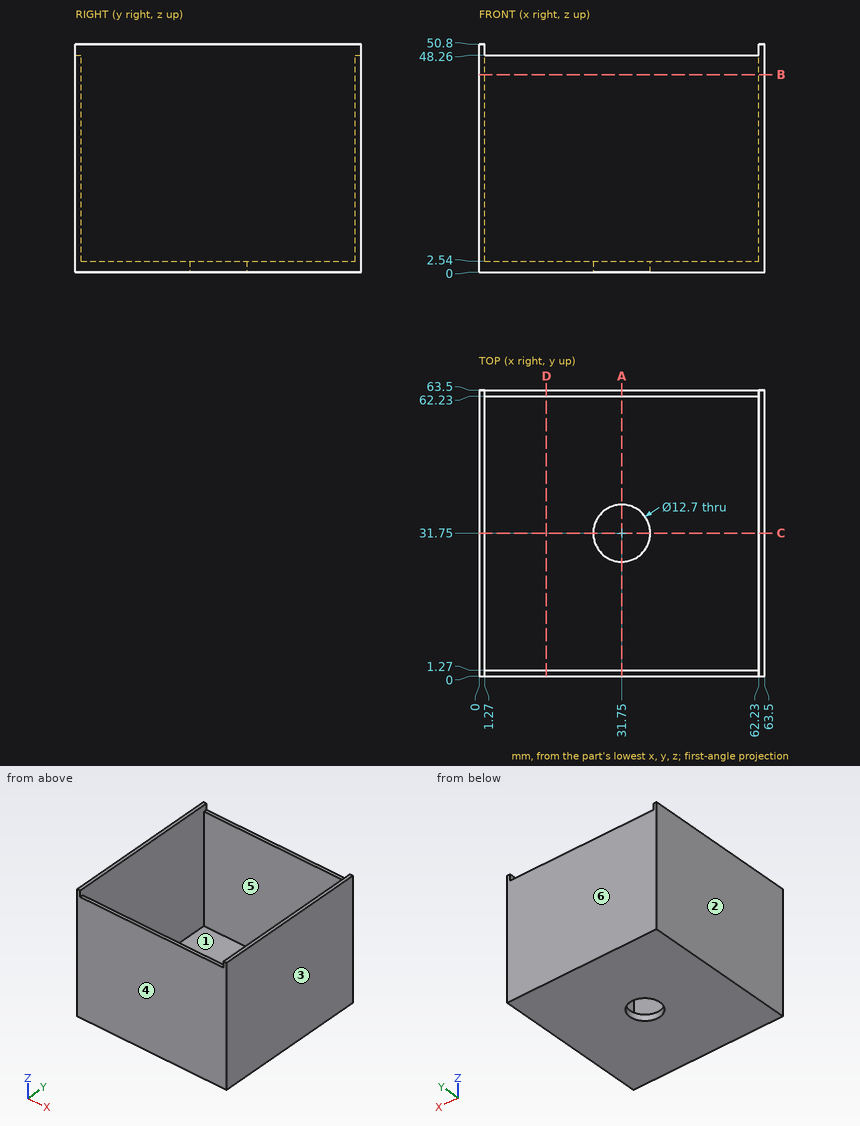
Job drawing, mm, ordinate dimensions from the low corner. One solid piece. A direction names the side the tool comes from. Coordinates: 2 decimals unless noted, no trailing zeros. Order: outer loops, then holes, each group sorted by start corner. A loop starts at its lowest first (then second) coordinate and runs counter-clockwise, first axis right, second up. Notation, with made-up numbers: (79, 38.25) - (91, 38.25) arc R22 ccw to (91, 74.25) - close; hole circle Ø6 at (50, 11). An arc over 180 degrees is marked (long way). Return JSON: item names as keys, results as strings. Group by question number.
1) Saw through at C-C, the plane y = 31.75. Write the cut outline in (x, z), plus the area to 3 significant figures.
2) Flat gauge pins, fed straight in: P1, Ø1, axis at x = 39.5, y = 0.5, coming from the +Z side; P2, Ø1.5, axis at x = 39, y = 15.5, coming from the +Z side; P3, Ø10, axis at x = 31.75, y = 31.75, coming from the +Z side. Where does each tip first touch, or does it go through?
3) Probe line 1 (Y direction, x = 7, z = 45.5); line 2 (Y direction, x = 31.75, z = 2.05). List the from-to ranges inside material, lowest first. Write a range as from..to.
4) Saw through at B-B, the plane z = 44. Write the cut outline in (x, y).
5) Mould opens along X. For the marked faces 1, 2, 3 and 4 say: released by +X, released by -X, zero draft, split by the parting line, or undercut.
6) Saw through at D-D, the plane x = 15. Write the cut outline in (y, z).
7) Saw through at A-A, the plane x = 31.75. Write the cut outline in (y, z).
8) Tool access for the marked faces 5 and 6: list every direction of +Z, -Z, +X, -X, +Y, -Y with a clear straight run to the whole face (end or side of a thin tool).
Values found:
{
 "1": {"outline": "(0, 0) - (25.4, 0) - (25.4, 2.54) - (1.27, 2.54) - (1.27, 50.8) - (0, 50.8) - close; (38.1, 0) - (63.5, 0) - (63.5, 50.8) - (62.23, 50.8) - (62.23, 2.54) - (38.1, 2.54) - close", "area": "252 mm²"},
 "2": {"P1": "stops at z = 48.26", "P2": "stops at z = 2.54", "P3": "passes through"},
 "3": {"line 1": "y = 0..1.27, 62.23..63.5", "line 2": "y = 0..25.4, 38.1..63.5"},
 "4": {"outline": "(0, 0) - (63.5, 0) - (63.5, 63.5) - (0, 63.5) - close; hole (1.27, 1.27) - (62.23, 1.27) - (62.23, 62.23) - (1.27, 62.23) - close"},
 "5": {"face 1": "undercut", "face 2": "released by -X", "face 3": "released by +X", "face 4": "zero draft"},
 "6": {"outline": "(0, 0) - (63.5, 0) - (63.5, 48.26) - (62.23, 48.26) - (62.23, 2.54) - (1.27, 2.54) - (1.27, 48.26) - (0, 48.26) - close"},
 "7": {"outline": "(0, 0) - (25.4, 0) - (25.4, 2.54) - (1.27, 2.54) - (1.27, 48.26) - (0, 48.26) - close; (38.1, 0) - (63.5, 0) - (63.5, 48.26) - (62.23, 48.26) - (62.23, 2.54) - (38.1, 2.54) - close"},
 "8": {"face 5": "+Z", "face 6": "+Z, -Z, +X, -X, +Y"}
}
